Input: part model. Units: mm. Frame: model coordinates. Face numbers are marked on the shaded views. A direction names the side the tool comes from. Coordinates: 2 decimals unless noted, no trailing zeros. Write each loop counter-clockwise with the first axis right and the second up, starting at its lowest first coordinate (ties: lowest second). Pieces come first, ordered by that corner, then holes.
1) Pin query (flat end, axial travel): pin 1 Ø8 at (y, z) = (39.5, 42) entering from +X; pin 2 Ø4 at (y, z) = (47, 34.5) entering from -X; pin 3 Ø6.5 at (x, z) = (5, 31) entering from +Y. Return the tip coordinate at first contact, or that it passes through.
2) Draft query along Y for the marked faces 4, 5 and 6. Return one class per face: pulls with the +Y half, pulls with the -Y half, needs draft (parallel to the pull), parting line crosses it, or undercut.
3) Section query C-C (y = 37). Output: boundary loops of the cut face in (x, z).
4) Section query B-B (z = 14.5). Output: boundary loops of the cut face in (x, y), then the cut area to 3 significant figures.
5) Section query A-A (x = 45). Output: boundary loops of the cut face in (y, z).
6) Section query D-D (z = 39). Output: boundary loops of the cut face in (x, y).
7) Set-up query: the marked faces 1, 2 and 3. Return all of +Z, -Z, +X, -X, +Y, -Y with unobstructed straight access to the full face (end or side cutting, diameter ignored); none if empty.
8) Line query: L1, parallel to Y at x = 40, z = 20; L2, parallel to X at y = 16, z = 35; L3, parallel to X at y = 47, z = 21. Output: solid intervals per line, ascending.
from build123d import *

# Parameters (mm, degrees)
F0_W     = 50.8
F0_H     = 50.8
F1_DEPTH = 50.8
F2_W     = 12.7
F2_H     = 12.7
F2_H_2   = 25.4
F3_DEPTH = 76.2
F5_DEPTH = 101.6


with BuildPart() as f1:
    # F0 (on Front) → F1 (new body)
    with BuildSketch(Plane.XZ):
        with Locations((25.4, 25.4)):
            Rectangle(F0_W, F0_H)
    extrude(amount=-F1_DEPTH)

    # F2 (on face) → F3 (cut)
    with BuildSketch(Plane.XY.offset(50.8)):
        with Locations((6.35, 44.45)):
            Rectangle(F2_W, F2_H)
        with Locations((6.35, 6.35)):
            Rectangle(F2_W, F2_H)
        with Locations((44.45, 25.4)):
            Rectangle(F2_W, F2_H_2)
    extrude(amount=-F3_DEPTH, mode=Mode.SUBTRACT)

    # F4 (on face) → F5 (cut)
    with BuildSketch(Plane.XZ):
        Polygon((50.8, 50.8), (25.4, 50.8), (50.8, 25.4), align=None)
    extrude(amount=-F5_DEPTH, mode=Mode.SUBTRACT)


solid = f1.part
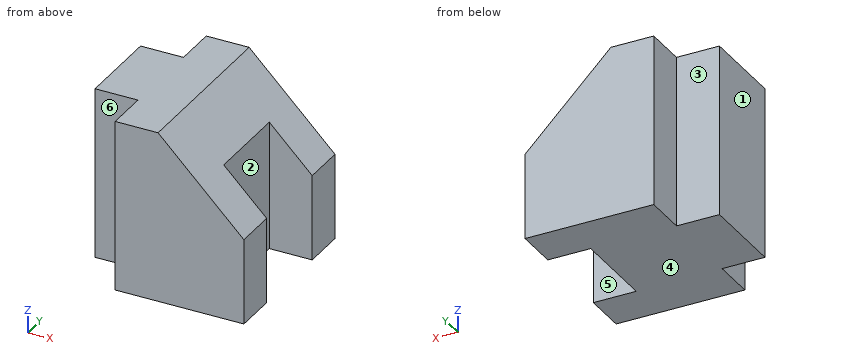
Answer:
1. pin 1: stops at x = 38.2
1. pin 2: stops at x = 12.7
1. pin 3: stops at y = 38.1
2. face 4: needs draft
2. face 5: undercut
2. face 6: pulls with the -Y half
3. outline: (0, 0) - (38.1, 0) - (38.1, 38.1) - (25.4, 50.8) - (0, 50.8) - close
4. outline: (0, 12.7) - (12.7, 12.7) - (12.7, 0) - (50.8, 0) - (50.8, 12.7) - (38.1, 12.7) - (38.1, 38.1) - (50.8, 38.1) - (50.8, 50.8) - (12.7, 50.8) - (12.7, 38.1) - (0, 38.1) - close
4. area: 1,940 mm2
5. outline: (0, 0) - (12.7, 0) - (12.7, 31.2) - (0, 31.2) - close; (38.1, 0) - (50.8, 0) - (50.8, 31.2) - (38.1, 31.2) - close
6. outline: (0, 12.7) - (12.7, 12.7) - (12.7, 0) - (37.2, 0) - (37.2, 50.8) - (12.7, 50.8) - (12.7, 38.1) - (0, 38.1) - close
7. face 1: +Z, -Z, -X, +Y, -Y
7. face 2: +Z, -Z, +X
7. face 3: +Z, -Z, -X, +Y
8. L1: y = 0 to 12.7, 38.1 to 50.8
8. L2: x = 0 to 38.1
8. L3: x = 12.7 to 50.8
